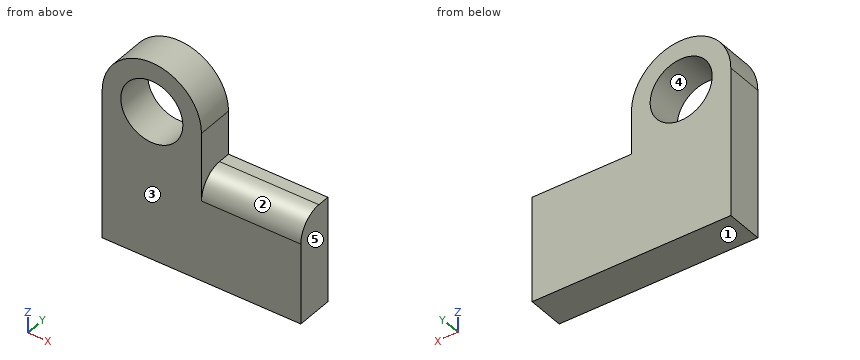
```python
from build123d import *

# Parameters (mm, degrees)
F1_DEPTH = 38.1
F2_R     = 25.4
F3_R     = 31.75
F4_DEPTH = 50.8


with BuildPart() as f1:
    # F0 (on Front) → F1 (new body)
    with BuildSketch(Plane.XZ):
        with BuildLine():
            ThreePointArc((-27.599881, 62.391328), (-78.399881, 113.191328), (-129.199881, 62.391328))
            Line((-129.199881, 62.391328), (-129.199881, -90.008672))
            Line((-129.199881, -90.008672), (74.000119, -90.008672))
            Line((74.000119, -90.008672), (74.000119, 17.941328))
            Line((74.000119, 17.941328), (-27.599881, 17.941328))
            Line((-27.599881, 17.941328), (-27.599881, 62.391328))
        make_face()
    extrude(amount=F1_DEPTH)

    # F2
    f2_edges = [f1.edges().sort_by_distance(p)[0] for p in [
        (23.200119, -38.1, 17.941328),
    ]]
    fillet(f2_edges, radius=F2_R)

    # F3 (on face) → F4 (cut)
    with BuildSketch(Plane.XZ.offset(38.1)):
        with Locations((-78.399881, 62.391328)):
            Circle(F3_R)
    extrude(amount=-F4_DEPTH, mode=Mode.SUBTRACT)


solid = f1.part
```
Geometry check sheet. Reference: the model listing, model coordinates, mm. Face numbers are marked on the shaded views. A direction names the side the tool comes from. Coordinates: 2 decimals unless noted, no trailing zeros. Loops run counter-clockwise (first coordinate to the right, second up) from the corner with the lowest first, then second, coordinate; pieces in that order, holes last.
Item 1: Sectioned sample at C-C, the plane z = 59.5. Record the boundary of the cut face in (x, y), then the cut area to 3 significant figures.
Item 2: Go/stop test with flat-tipped pins: pin 1 Ø5 at (y, z) = (-24, 19) entering from +X; pin 2 Ø14 at (x, y) = (7.5, -5.5) entering from +Z; pin 3 Ø5 at (x, z) = (15, 14.5) entering from -Y. Record where each tip stops, or that it passes through.
Item 3: Sectioned sample at D-D, the plane x = -14. Record the boundary of the cut face in (y, z), then the cut area to 3 significant figures.
Item 4: Access from +Z, -Z, +X, -X, +Y, -Y to the whole of each face (thin tool, end or side, straight path). Record for the marked faces 1 and 2.
Item 5: Sectioned sample at A-A, the plane x = -59. Record the boundary of the cut face in (y, z).
Item 6: Sectioned sample at B-B, the plane y = -7.5. Record the boundary of the cut face in (x, z).
Item 7: Thickness scan on line 1 (X direction, y = -6.5, z = 20.5); line 2 (X direction, y = -20, z = 35); line 3 (X direction, y = -27.5, z = 71). Record the ranges inside material, lowest first.
Item 8: Release check for a two-part mould opening along X. For the marked faces 3, 4 and 5 record: released by +X, released by -X, zero draft, split by the parting line, or undercut.
Check result:
1. outline: (-129.2, -38.1) - (-110.02, -38.1) - (-110.02, 0) - (-129.2, 0) - close; (-46.78, -38.1) - (-27.6, -38.1) - (-27.6, 0) - (-46.78, 0) - close
1. area: 1,460 mm2
2. pin 1: stops at x = -27.6
2. pin 2: stops at z = 17.94
2. pin 3: stops at y = -29.03
3. outline: (-38.1, -90.01) - (0, -90.01) - (0, 17.94) - (-12.7, 17.94) arc R25.4 ccw to (-38.1, -7.46) - close
3. area: 3,970 mm2
4. face 1: -Z, +X, -X, +Y, -Y
4. face 2: +Z, +X, -Y
5. outline: (-38.1, -90.01) - (0, -90.01) - (0, 37.26) - (-38.1, 37.26) - close; (-38.1, 87.53) - (0, 87.53) - (0, 109.34) - (-38.1, 109.34) - close
6. outline: (-129.2, -90.01) - (74, -90.01) - (74, 17.94) - (-27.6, 17.94) - (-27.6, 62.39) arc R50.8 ccw to (-129.2, 62.39) - close; hole circle Ø63.5 at (-78.4, 62.39)
7. line 1: x = -129.2 to -27.6
7. line 2: x = -129.2 to -94.46, -62.34 to -27.6
7. line 3: x = -128.47 to -108.96, -47.84 to -28.33
8. face 3: zero draft
8. face 4: undercut
8. face 5: released by +X
